from build123d import *

# Parameters (mm, degrees)
F0_W     = 63.5
F0_H     = 38.1
F1_DEPTH = 20.32
F3_D     = 6.7564


with BuildPart() as f1:
    # F0 (on Front) → F1 (new body)
    with BuildSketch(Plane.XZ):
        with Locations((31.75, 19.05)):
            Rectangle(F0_W, F0_H)
    extrude(amount=-F1_DEPTH)

    # F3 (through all)
    with Locations(Plane.XZ):
        with Locations((9.525, 19.05), (53.975, 19.05)):
            Hole(F3_D / 2)


solid = f1.part
Work out the finished part from the listing and answer in its coordinate system (mm). Coordinates: 2 decimals unless noted, no trailing zeros. Order: outer loops, then holes, each group sorted by start corner. A loop starts at its lowest first (then second) coordinate and runs counter-clockwise, first axis right, second up. Notation, with made-up numbers: (-6.75, -8) - (23.25, -8) arc R22 cw to (23.25, 22) - close; hole circle Ø11 at (-40, -21.5). An arc over 180 degrees is marked (long way). Put each result on its own line as item: value. Start each with the question number.
1) A flat-ended cylindrical pin translates along its axis: pin 1 (4 mm diameter, centred on x = 53.975, z = 19.05, fed in from +Y). Find the tip coordinate at first contact, or state that the pin passes through.
2) Find the intervals of material crossed by line 1 (Z direction, x = 54, y = 18.5); line 2 (X direction, y = 6.75, z = 16); line 3 (Z direction, x = 52.5, y = 10.5), in increasing order. Write a range as from..to.
3) Find section B-B (y = 15.75). Give the vertices of the cut face in (x, z) (3 decimals).
4) Find section A-A (z = 19.05). Give the vertices of the cut face in (x, y), plus the area to 3 significant figures.
5) Find section C-C (x = 7.5). Give the vertices of the cut face in (y, z).
6) For a pull along Z with two mould halves and no side action, classify faces 1 (the flat face through (31, 10, 0)), 2 (the cylindrical face through (57.35, 10.3, 19.2)), 3 (the flat face through (63.5, 10, 19)) as released by +Z, released by -Z, zero draft, split by the parting line, or undercut.
Results list:
1. pin 1: passes through
2. line 1: z = 0..15.67, 22.43..38.1
2. line 2: x = 0..8.07, 10.98..52.52, 55.43..63.5
2. line 3: z = 0..16.01, 22.09..38.1
3. outline: (0, 0) - (63.5, 0) - (63.5, 38.1) - (0, 38.1) - close; hole circle Ø6.756 at (9.525, 19.05); hole circle Ø6.756 at (53.975, 19.05)
4. outline: (0, 0) - (6.15, 0) - (6.15, 20.32) - (0, 20.32) - close; (12.9, 0) - (50.6, 0) - (50.6, 20.32) - (12.9, 20.32) - close; (57.35, 0) - (63.5, 0) - (63.5, 20.32) - (57.35, 20.32) - close
4. area: 1,020 mm^2
5. outline: (0, 0) - (20.32, 0) - (20.32, 16.35) - (0, 16.35) - close; (0, 21.75) - (20.32, 21.75) - (20.32, 38.1) - (0, 38.1) - close
6. face 1: released by -Z
6. face 2: undercut
6. face 3: zero draft
